Build history of the part. All positions in model axes, mm. A direction names the side the tool comes from. Give positions to 0.01 mm unless a question says otherwise; leave off trailing zeros. Write each loop counter-clockwise with the first axis right and the second up, starting at its lowest first coordinate (ties: lowest second). Pieces come first, ordered by that corner, then holes. Notation, with made-up numbers: (63.25, 18.25) - (87.25, 18.25) arc R9 ccw to (87.25, 26.25) - close; hole circle Ø3 at (57.25, 74). An arc over 180 degrees is marked (long way). Use one line per item in the form item = value. Start each with the question number.
Autodesk Inventor part; units mm, degrees
ref_plane "YZ Plane" through (0, 0, 0) normal (1, 0, 0) x (0, 1, 0)
ref_plane "XZ Plane" through (0, 0, 0) normal (0, 1, 0) x (-1, 0, 0)
ref_plane "XY Plane" through (0, 0, 0) normal (0, 0, 1) x (1, 0, 0)
sketch "Sketch1" plane through (0, 0, 0) normal (0, 0, 1) x (1, 0, 0)
  circle A0 centre (0, 35.5) radius 10 construction
  line L0 (-2.9, -10) -> (-2.9, 0)
  line L1 (-2.9, 0) -> (2.9, 0)
  line L2 (2.9, 0) -> (2.9, -10)
  line L3 (-3.3173, -10) -> (-2.9, -10)
  line L4 (2.9, -10) -> (3.3173, -10)
  circle A1 centre (-7.0711, 28.4289) radius 1.25
  circle A2 centre (7.0711, 28.4289) radius 1.25
  circle A3 centre (0, 45.5) radius 1.25
  line L5 (-16, 37) -> (-16, 43)
  line L6 (16, 37) -> (16, 43)
  line L7 (-5.2638, -8.4597) -> (-16, 37)
  line L8 (5.2638, -8.4597) -> (16, 37)
  line L9 (-16, 43) -> (-4.8446, 48.5777)
  line L10 (-3.0557, 49) -> (3.0557, 49)
  line L11 (4.8446, 48.5777) -> (16, 43)
  arc A4 (-3.0557, 49) -> (-4.8446, 48.5777) centre (-3.0557, 45) ccw
  arc A5 (4.8446, 48.5777) -> (3.0557, 49) centre (3.0557, 45) ccw
  line L12 (0, 49) -> (0, 0) construction
  line L13 (-7.0711, 28.4289) -> (0, 35.5) construction
  line L14 (0, 35.5) -> (7.0711, 28.4289) construction
  arc A6 (-5.2638, -8.4597) -> (-3.3173, -10) centre (-3.3173, -8) ccw
  arc A7 (3.3173, -10) -> (5.2638, -8.4597) centre (3.3173, -8) ccw
  circle A8 centre (0, 35.5) radius 15.25 construction
  point P0 (0, 43)
  point P1 (4.9, -10)
  point P2 (-4.9, -10)
  point P3 (0, 43)
  point P4 (-4, 49)
  point P5 (4, 49)
  dimension "d69" = 20
  dimension "d88" = 5.8
  dimension "d95" = 2
  dimension "d96" = 2
  dimension "d97" = 10
  dimension "d98" = 10
  dimension "d109" = 43
  dimension "d112" = 2.5
  dimension "d113" = 2.5
  dimension "d114" = 2.5
  dimension "d123" = 32
  dimension "d126" = 8
  dimension "d127" = 4
  dimension "d144" = 16
  dimension "d145" = 35.5
  dimension "d153" = 6
  dimension "d155" = 6
  dimension "d156" = 135
  dimension "d163" = 2
  dimension "d169" = 30.5
extrude "Extrusion7" add sketch "Sketch1" along normal blind 6
sketch "Sketch3" plane through (0, 0, 6) normal (0, 0, 1) x (1, 0, 0)
  line L0 (16, 37) -> (16, 43)
  line L1 (-16, 43) -> (-16, 37)
  line L2 (-10, 43) -> (10, 43)
  line L3 (10, 43) -> (10, 37)
  line L4 (-10, 37) -> (-10, 43)
  line L5 (10, 37) -> (5, 37)
  line L6 (-5, 37) -> (-10, 37)
  line L7 (5.2638, -8.4597) -> (16, 37)
  line L8 (-16, 37) -> (-5.2638, -8.4597)
  circle A0 centre (0, 45.5) radius 1.25
  circle A1 centre (7.0711, 28.4289) radius 1.25
  circle A2 centre (-7.0711, 28.4289) radius 1.25
  line L9 (3.0557, 49) -> (-3.0557, 49)
  line L10 (0, 45.5) -> (0, 35.4997) construction
  line L11 (-7.0711, 28.4289) -> (0, 35.5003) construction
  line L12 (7.0711, 28.4289) -> (0, 35.4997) construction
  line L13 (-5, 37) -> (-3.5355, 30.7988)
  line L14 (-3, 26.2019) -> (-3, 20)
  line L15 (-1, 18) -> (1, 18)
  line L16 (3, 20) -> (3, 26.2019)
  line L17 (3.5355, 30.7988) -> (5, 37)
  arc A3 (-3, 26.2019) -> (-3.5355, 30.7988) centre (-23, 26.2019) ccw
  arc A4 (3.5355, 30.7988) -> (3, 26.2019) centre (23, 26.2019) ccw
  arc A5 (-3, 20) -> (-1, 18) centre (-1, 20) ccw
  arc A6 (1, 18) -> (3, 20) centre (1, 20) ccw
  point P0 (0, 0)
  point P1 (4.9, -10)
  point P2 (-4.9, -10)
  point P3 (0, 18)
  dimension "d132" = 6
  dimension "d134" = 6
  dimension "d135" = 6
  dimension "d148" = 5
  dimension "d149" = 5
  dimension "d157" = 25
  dimension "d160" = 6
  dimension "d161" = 20
  dimension "d162" = 2
extrude "Extrusion8" cut sketch "Sketch3" against normal through all contours L2 L3 L5 L17 A4 L16 A6 L15 A5 L14 A3 L13 L6 L4
properties part number "Vert Moto Mount skinny"
(1) Cut at B-B, the plane x = 0. Give the cut face in (y, z).
(2) Wall check: line 1 (Y direction, x = 0, z = 1.7); line 2 (Y direction, x = -1, z = 5.6); line 3 (X direction, y = 34, z = 1.2). Give the ranges that are in metal, low to high. Write a range as from..to.
(3) Cut at D-D, the plane y = 38. Give the cut face in (x, z).
(4) Which spindle directions (+Z, -Z, +X, -X, +Y, -Y) get a long thin tool onto all of the face, cutting with end or side? Do faces 1 (the cylindrical face through (3.14, 28.55, 3.04)), 2 (the flat face through (-16, 40, 3)), 3 (the flat face through (0, 0, 3)). Say none if no direction does.
(5) Pin check, flat tips, straight feed: pin 1 Ø1.5 at (y, z) = (12.5, 1) entering from -X; pin 2 Ø2 at (x, z) = (-11, 5.5) entering from +Y; pin 3 Ø3 at (y, z) = (22, 3.5) entering from -X; pin 4 Ø6 at (x, y) = (-12.5, 11.5) entering from -Z. Stop position of each tip, or through.
(6) Two-plate mould, pull along X, no slides. Class faces 4 (the flat face through (10.557, 13.952, 2.958)), 5 (the flat face through (-10.557, 13.952, 2.958)), 6 (the flat face through (10, 40, 3)): +X half, -X half, draft (parallel to the pull), parting line (faces both ways), or undercut.
(7) Cut at A-A, the plane y = 45.5. Give the cut face in (x, z).
(8) Cut at C-C, the plane z = 0.9. State how many separate pieces and enclosed holes the cut face has, then the cut area to 3 significant figures.
Solution:
q1.outline = (0, 0) - (18, 0) - (18, 6) - (0, 6) - close; (43, 0) - (44.25, 0) - (44.25, 6) - (43, 6) - close; (46.75, 0) - (49, 0) - (49, 6) - (46.75, 6) - close
q2.line_1 = 0..18, 43..44.25, 46.75..49
q2.line_2 = 0..18, 43..44.75, 46.25..49
q2.line_3 = -15.29..-4.29, 4.29..15.29
q3.outline = (-16, 0) - (-10, 0) - (-10, 6) - (-16, 6) - close; (10, 0) - (16, 0) - (16, 6) - (10, 6) - close
q4.face_1 = +Z, -Z
q4.face_2 = +Z, -Z, -X, +Y, -Y
q4.face_3 = +Z, -Z, -Y
q5.pin_1 = -10.39
q5.pin_2 = 46
q5.pin_3 = -12.81
q5.pin_4 = 0
q6.face_4 = +X half
q6.face_5 = -X half
q6.face_6 = undercut
q7.outline = (-11, 0) - (-1.25, 0) - (-1.25, 6) - (-11, 6) - close; (1.25, 0) - (11, 0) - (11, 6) - (1.25, 6) - close
q8.separate_pieces = 1
q8.enclosed_holes = 4
q8.area = 971 mm2
